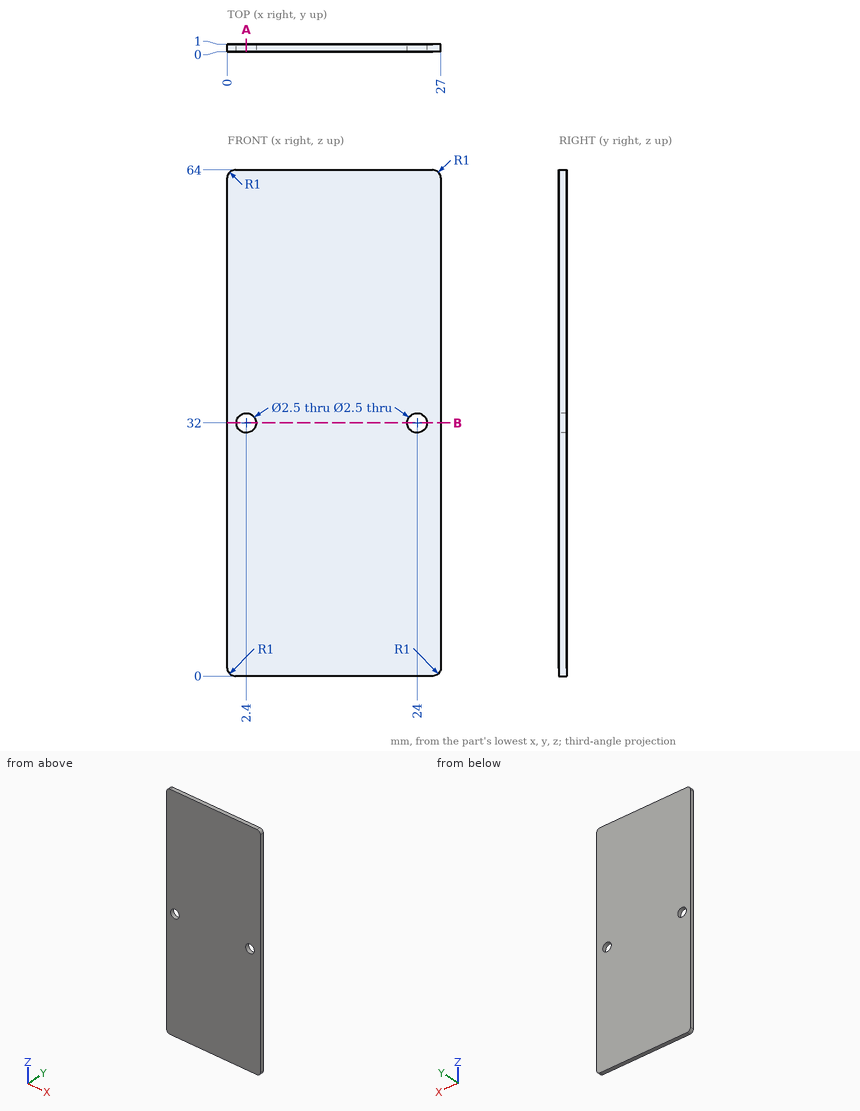
The drawing under review shows one solid part. Ordinate dimensions are in mm from its lowest x, y, z. Coordinates: 2 decimals unless noted, no trailing zeros. Write each loop counter-clockwise with the first axis right and the second up, starting at its lowest first coordinate (ties: lowest second). Pieces come first, ordered by that corner, then holes.
1) Add section A-A (x = 2.4). Write out the cut boundary in (y, z).
2) Add section B-B (z = 32). Write out the cut boundary in (x, y).
3) To check wall thickness, follow L1, parallel to Z at x = 2.4, y = 0.7; L2, parallel to Z at x = 23, y = 0.3. State the ranges of each line that lie inside material, in increasing order.
4) Insertion check: pin 1 (3 mm diameter, centred on x = 2.4, z = 32, fed in from -Y); pin 2 (1.5 mm diameter, centred on x = 24, z = 32, fed in from -Y). Each pin has a flat end and moves straight along its axis. Give the tip position at first contact, or say it passes through.
Check result:
1. outline: (0, 0) - (1, 0) - (1, 30.75) - (0, 30.75) - close; (0, 33.25) - (1, 33.25) - (1, 64) - (0, 64) - close
2. outline: (0, 0) - (1.15, 0) - (1.15, 1) - (0, 1) - close; (3.65, 0) - (22.75, 0) - (22.75, 1) - (3.65, 1) - close; (25.25, 0) - (27, 0) - (27, 1) - (25.25, 1) - close
3. L1: z = 0 to 30.75, 33.25 to 64
3. L2: z = 0 to 31.25, 32.75 to 64
4. pin 1: stops at y = 0
4. pin 2: passes through
